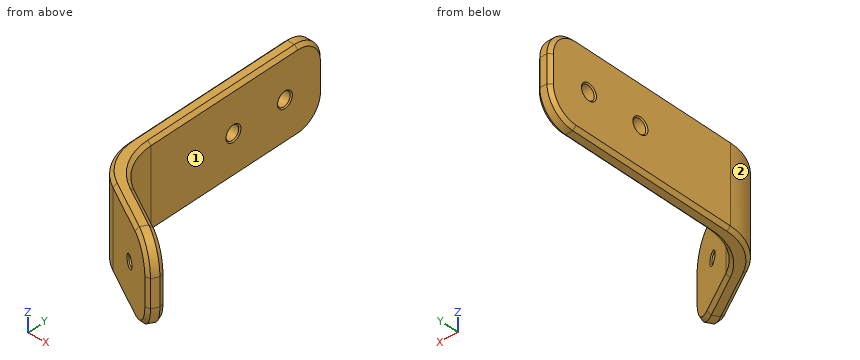
from build123d import *

# Parameters (mm, degrees)
SKETCH2_W                       = 3.175
SKETCH2_H                       = 19.05
F_1_8_0_125_DIAMETER_HOLE1_D    = 3.175
F_3_32_0_09375_DIAMETER_HOLE2_D = 2.38125
FILLET1_R                       = 12.7
FILLET2_R                       = 6.35
CHAMFER3_SIZE                   = 0.762
CHAMFER2_SIZE                   = 0.254


with BuildPart() as part:
    # Sweep1: sweep along a path in Sketch1
    with BuildLine(Plane.XY) as sweep1_path:
        Line((0, 0), (0, -31.75))
        Line((0, -31.75), (0, -50.8))
        Line((0, -50.8), (21.997045256, -63.5))
    # Sketch2 → Sweep1 (sweep)
    with BuildSketch(Plane(origin=(0, 0, 0), x_dir=(1, 0, 0), z_dir=(0, 1, 0))):
        Rectangle(SKETCH2_W, SKETCH2_H)
    sweep(path=sweep1_path.line, transition=Transition.RIGHT)

    # 1/8 (0.125) Diameter Hole1 (through all)
    with Locations(Plane(origin=(1.5875, 0, 0), x_dir=(0, 0, -1), z_dir=(1, 0, 0))):
        with Locations((0, -9.525), (0, -22.225)):
            Hole(F_1_8_0_125_DIAMETER_HOLE1_D / 2)

    # 3/32 (0.09375) Diameter Hole2 (through all)
    with Locations(Plane(origin=(-21.203295256, -36.725184671, 0), x_dir=(0.866025404, -0.5, 0), z_dir=(0.5, 0.866025404, 0))):
        with Locations((41.275, 0)):
            Hole(F_3_32_0_09375_DIAMETER_HOLE2_D / 2)

    # Fillet1
    fillet1_edges = [part.edges().sort_by_distance(p)[0] for p in [
        (1.5875, -49.883456448, 0),
        (-1.5875, -51.716543552, 0),
    ]]
    fillet(fillet1_edges, radius=FILLET1_R)

    # Fillet2
    fillet2_edges = [part.edges().sort_by_distance(p)[0] for p in [
        (21.997045256, -63.5, -9.525),
        (21.997045256, -63.5, 9.525),
        (0, 0, -9.525),
        (0, 0, 9.525),
    ]]
    fillet(fillet2_edges, radius=FILLET2_R)

    # Chamfer3
    chamfer3_edges = [part.edges().sort_by_distance(p)[0] for p in [
        (10.233266971, -58.541266545, -9.525),
        (10.233266971, -58.541266545, 9.525),
        (12.614516971, -56.249907664, -9.525),
        (0.113977372, -50.734195134, -9.525),
        (0.113977372, -50.734195134, -9.525),
        (0.113977372, -50.734195134, 9.525),
        (12.614516971, -56.249907664, 9.525),
        (0.113977372, -50.734195134, 9.525),
        (3.288977372, -48.901108029, 9.525),
        (3.288977372, -48.901108029, 9.525),
        (3.288977372, -48.901108029, -9.525),
        (3.288977372, -48.901108029, -9.525),
        (1.5875, -24.450554014, 9.525),
        (1.5875, -24.450554014, -9.525),
        (-1.5875, -25.367097567, -9.525),
        (-1.5875, -25.367097567, 9.525),
        (21.203295256, -64.874815329, 0),
        (19.592598909, -63.944879359, 7.665128061),
        (19.592598909, -63.944879359, -7.665128061),
        (22.790795256, -62.125184671, 0),
        (21.180098909, -61.195248702, 7.665128061),
        (21.180098909, -61.195248702, -7.665128061),
        (1.5875, 0, 0),
        (-1.5875, 0, 0),
        (-1.5875, -25.367097567, 9.525),
        (-1.5875, -25.367097567, -9.525),
        (-1.5875, -1.859871939, 7.665128061),
        (-1.5875, -1.859871939, -7.665128061),
        (1.5875, -24.450554014, -9.525),
        (1.5875, -24.450554014, 9.525),
        (1.5875, -1.859871939, 7.665128061),
        (1.5875, -1.859871939, -7.665128061),
    ]]
    chamfer(chamfer3_edges, length=CHAMFER3_SIZE)

    # Chamfer2
    chamfer2_edges = [part.edges().sort_by_distance(p)[0] for p in [
        (1.5875, -22.225, -1.5875),
        (-1.5875, -22.225, -1.5875),
        (1.5875, -9.525, -1.5875),
        (-1.5875, -9.525, -1.5875),
        (13.985514781, -60.707627829, 0),
        (15.573014781, -57.957997171, 0),
    ]]
    chamfer(chamfer2_edges, length=CHAMFER2_SIZE)


solid = part.part
The listing builds one solid part. Answer for the finished solid, in the listing's coordinates (mm). Face numbers are marked on the shaded views. A direction names the side the tool comes from. Round coordinates to 2 decimals unless told otherwise and drop trailing zeros. Order: outer loops, then holes, each group sorted by start corner. A loop starts at its lowest first (then second) coordinate and runs counter-clockwise, first axis right, second up. Notation, with made-up numbers: (59.25, -33.75) -> (95.25, -33.75) arc R3 cw to (95.25, -28.75) -> close; hole circle Ø7 at (-28, 18). An arc over 180 degrees is marked (long way). Write each question's results on one line, items separated by ' | '. Start each with the question number.
Q1. Find section B-B (z = 0). Give the number of separate pieces and of enclosed holes in the cut face, then the cut area to 3 significant figures.
Q2. Straight lines are drawn through the part: probe 1 along Y at (x, z) = (-0.25, 0); probe 2 along Y at (x, z) = (0.65, 0); probe 3 along X at (y, z) = (-7, 8.25). For each, find the intervals that lie inside material, in ascending order. Write a range as from..to.
Q3. Each of these flat-tipped pins is pushed along its axis until it touches: pin 1 (9 mm diameter, centred on y = -23, z = 0, fed in from +X); pin 2 (4 mm diameter, centred on x = 6.5, z = 0.5, fed in from -Y). Where does it stop, or does it pass through?
Q4. Which of the six approach directions +Z, -Z, +X, -X, +Y, -Y give full straight-line access (tool end or side, diameter ignored) to the marked faces 1 and 2?
Q5. Find section A-A (y = -31.5). Determine the outline of the cut face in (x, z) (1 decimal).
Worked answers:
1) separate pieces: 4 | enclosed holes: 0 | area: 213 mm2
2) probe 1: y = -50.06..-23.81, -20.64..-11.11, -7.94..0 | probe 2: y = -51.58..-23.81, -20.64..-11.11, -7.94..0 | probe 3: x = -1.59..1.59
3) pin 1: stops at x = 1.59 | pin 2: stops at y = -57.54
4) face 1: +Z, -Z, +X, +Y | face 2: +Z, -Z, -X, -Y
5) outline: (-1.6, -8.8) -> (-0.8, -9.5) -> (0.8, -9.5) -> (1.6, -8.8) -> (1.6, 8.8) -> (0.8, 9.5) -> (-0.8, 9.5) -> (-1.6, 8.8) -> close
